Geometry: final body of the model. Coordinates: model frame, mm. Give positions to 0.01 mm unless a question says otherwise; leave off trailing zeros. Write each loop counter-clockwise with the first axis right and the second up, starting at its lowest first coordinate (ties: lowest second). Pieces come first, ordered by that corner, then holes. Notation, with made-up numbers: (39, 72.25) -> (44, 72.25) arc R30 ccw to (44, 99.25) -> close; hole circle Ø10 at (-21, 28). An arc over 180 degrees is marked (long way). Answer as a JSON object with one key per item and string values. Group by question number.
(1) Material intervals for probe 1 along Y at (x, z) = (13.5, 1.6); probe 2 along X at (y, z) = (-18.5, 1.15); probe 3 along Y at (x, z) = (6.5, 1.25), sorted ascending.
(2) Section query C-C on x = -10.5. Output: boundary loops of the cut face in (y, z).
(3) Section query B-B on y = -15. Output: boundary loops of the cut face in (x, z).
(4) Section query A-A on z = 3.65. Output: boundary loops of the cut face in (x, y), plus the area to 3 significant figures.
(5) Contact query for flat-ended pins moving along their axis: pin 1 Ø1 at (x, z) = (0.5, 1.5) entering from +Y; pin 2 Ø1.5 at (x, z) = (22.5, 1.5) entering from -Y; pin 3 Ø2.5 at (x, z) = (0, 2.5) entering from -Y. Output: stop coordinate, or through.
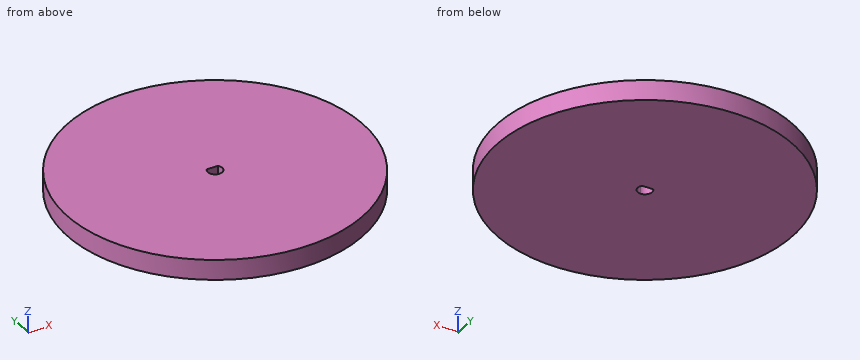
from build123d import *

# Parameters (mm, degrees)
F0_R     = 31.75
F1_DEPTH = 4.318
F3_DEPTH = 4.318


with BuildPart() as f1:
    # F0 (on Top) → F1 (new body)
    with BuildSketch(Plane.XY):
        Circle(F0_R)
    extrude(amount=F1_DEPTH)

    # F2 (on face) → F3 (cut, through all)
    with BuildSketch(Plane.XY.offset(4.318)):
        with BuildLine():
            ThreePointArc((0, -1.55), (1.096016, -1.096016), (1.55, 0))
            ThreePointArc((1.55, 0), (1.455699, 0.53239), (1.184272, 1))
            Line((1.184272, 1), (0, 1))
            Line((0, 1), (0, -1.55))
        make_face()
        with BuildLine():
            ThreePointArc((-1.184272, 1), (-1.405792, -0.652878), (0, -1.55))
            Line((0, -1.55), (0, 1))
            Line((0, 1), (-1.184272, 1))
        make_face()
    extrude(amount=-F3_DEPTH, mode=Mode.SUBTRACT)


solid = f1.part
Answer list:
{
 "1": {"probe 1": "-28.74 to 28.74", "probe 2": "-25.8 to 25.8", "probe 3": "-31.08 to 31.08"},
 "2": {"outline": "(-29.96, 0) -> (29.96, 0) -> (29.96, 4.32) -> (-29.96, 4.32) -> close"},
 "3": {"outline": "(-27.98, 0) -> (27.98, 0) -> (27.98, 4.32) -> (-27.98, 4.32) -> close"},
 "4": {"outline": "circle Ø63.5 at (0, 0); hole (-1.18, 1) arc R1.55 ccw to (0, -1.55) arc R1.55 ccw to (1.55, 0) arc R1.55 ccw to (1.18, 1) -> close", "area": "3,160 mm2"},
 "5": {"pin 1": "y = 31.75", "pin 2": "y = -23.13", "pin 3": "y = -31.75"}
}
